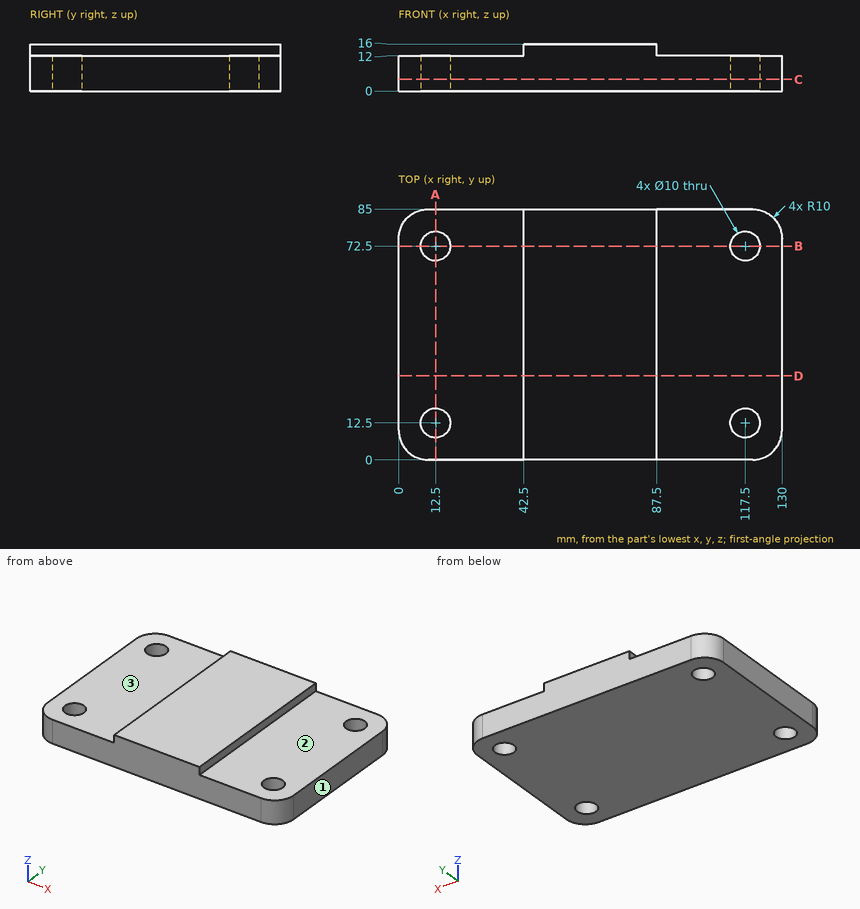
Input: dimensioned drawing with shaded views. Units: mm. Origin: part minimum x, y, z. A direction names the side the tool comes from. Round coordinates to 2 decimals unless told otherwise and drop trailing zeros. Loops run counter-clockwise (first coordinate to the right, second up) from the corner with the lowest first, then second, coordinate; pieces in that order, holes last. Notation, with made-up numbers: M 66.5,37.5 L 91.5,37.5 A14 ccw 91.5,43.5 Z; hole C 57.5,-27 d2. An arc over 180 degrees is marked long. Return JSON: item names as keys, results as strings. Group by question number.
1. Section query D-D on y = 28.5. Output: boundary loops of the cut face in (x, z).
2. Section query C-C on z = 4. Output: boundary loops of the cut face in (x, y).
3. Section query A-A on x = 12.5. Output: boundary loops of the cut face in (y, z), and give its area (3 significant figures).
4. Section query B-B on y = 72.5. Output: boundary loops of the cut face in (x, z), and give its area (3 significant figures).
5. Reachability of the marked faces 1, 2 and 3 from +Z, -Z, +X, -X, +Y, -Y: full face, straight path, thin tool, end or side. Return the list, or none.
6. Material intervals for line 1 along Y through (x, z) = (12.5, 7); line 2 along X through (y, z) = (12, 6.75); line 3 along Y through (x, z) = (11, 5.75), sorted ascending. Write a range as from..to.
7. Pin query (flat end, axial travel): pin 1 (16 mm diameter, centred on x = 12.5, y = 72.5, fed in from +Z); pin 2 (9 mm diameter, centred on x = 117.5, y = 12.5, fed in from +Z). Return the tip coordinate at first contact, or that it passes through.
Checks:
{
 "1": {"outline": "M 0,0 L 130,0 L 130,12 L 87.5,12 L 87.5,16 L 42.5,16 L 42.5,12 L 0,12 Z"},
 "2": {"outline": "M 0,10 A10 ccw 10,0 L 120,0 A10 ccw 130,10 L 130,75 A10 ccw 120,85 L 10,85 A10 ccw 0,75 Z; hole C 12.5,12.5 d10; hole C 12.5,72.5 d10; hole C 117.5,12.5 d10; hole C 117.5,72.5 d10"},
 "3": {"outline": "M 0,0 L 7.5,0 L 7.5,12 L 0,12 Z; M 17.5,0 L 67.5,0 L 67.5,12 L 17.5,12 Z; M 77.5,0 L 85,0 L 85,12 L 77.5,12 Z", "area": "780 mm²"},
 "4": {"outline": "M 0,0 L 7.5,0 L 7.5,12 L 0,12 Z; M 17.5,0 L 112.5,0 L 112.5,12 L 87.5,12 L 87.5,16 L 42.5,16 L 42.5,12 L 17.5,12 Z; M 122.5,0 L 130,0 L 130,12 L 122.5,12 Z", "area": "1,500 mm²"},
 "5": {"face 1": "+Z, -Z, +X, +Y, -Y", "face 2": "+Z, +X, +Y, -Y", "face 3": "+Z, -X, +Y, -Y"},
 "6": {"line 1": "y = 0..7.5, 17.5..67.5, 77.5..85", "line 2": "x = 0..7.53, 17.47..112.53, 122.47..130", "line 3": "y = 0..7.73, 17.27..67.73, 77.27..85"},
 "7": {"pin 1": "stops at z = 12", "pin 2": "passes through"}
}
